Check sheet for the modelled part. Datum: model origin and axes. Units: mm. A direction names the side the tool comes from. Round coordinates to 2 decimals unless told otherwise and drop trailing zeros. Loops run counter-clockwise (first coordinate to the right, second up) from the corner with the lowest first, then second, coordinate; pieces in that order, holes last. Notation, with made-up numbers: (2, -13.75) -> (30, -13.75) arc R10 ccw to (30, 5.25) -> close; hole circle Ø4 at (62.5, -29). An arc over 180 degrees is marked (long way). One line per item, written item: value. Start each with the question number.
1. Material ranges on L1, parallel to X at y = 3.75, z = 1.4; L2, parallel to Y at x = 3.5, z = 1.75; L3, parallel to Y at x = 5, z = 4.8, recorded low to high.
2. Cross-section at C-C on y = 3. Record the cut outline in (x, z), then the cut area to 3 significant figures.
3. Release check for a two-part mould opening along X. For faces 6 (the face through (7, 2.25, 5)), 7 (the face through (0.301, 3.465, 5.715)), 8 (the face through (7, 0, 2)) record: +X half, -X half, draft (parallel to the pull), parting line (faces both ways), or undercut.
4. Cross-section at B-B on x = 11. Record the cut outline in (y, z).
5. Cross-section at D-D on x = 2.5. Record the cut outline in (y, z), then the cut area to 3 significant figures.
6. Cross-section at A-A on z = 2.85. Record the cut outline in (x, y), then the cut area to 3 significant figures.
7. Set-up check for faces 1 (the face through (6.9, 3.75, 3.5)), 2 (the face through (13.699, 0.285, 2.535)), 3 (the face through (8.5, 6.5, 0.5)), 4 (the face through (1.67, 3, 5)), 5 (the face through (13, 3, 1)): record each of +Z, -Z, +X, -X, +Y, -Y from which the full face is reachable in a straight line by a thin tool's end or side.
8. Go/stop test with a flat-tipped pin: pin 1 (1.2 mm diameter, centred on x = 8.5, y = 3.5, fed in from +Z). Record where the tip stops, or that it passes through.
Autodesk Inventor part; units mm, degrees
ref_plane "YZ Plane" through (0, 0, 0) normal (1, 0, 0) x (0, 1, 0)
ref_plane "XZ Plane" through (0, 0, 0) normal (0, 1, 0) x (-1, 0, 0)
ref_plane "XY Plane" through (0, 0, 0) normal (0, 0, 1) x (1, 0, 0)
sketch "Sketch1" plane through (0, 0, 0) normal (0, 0, 1) x (1, 0, 0)
  line L0 (0, 0) -> (14, 0)
  line L1 (14, 0) -> (14, 7)
  line L2 (14, 7) -> (0, 7)
  line L3 (0, 7) -> (0, 0)
  dimension "d2" = 14
  dimension "d3" = 7
extrude "Extrusion1" add sketch "Sketch1" along normal blind 6
sketch "Sketch2" plane through (0, 0, 6) normal (0, 0, 1) x (1, 0, 0)
  line L0 (0, 7) -> (14, 0) construction
  line L1 (0, 0) -> (14, 7) construction
  line L2 (1.67, 4.75) -> (12.33, 4.75)
  line L3 (12.33, 4.75) -> (12.33, 2.25)
  line L4 (12.33, 2.25) -> (1.67, 2.25)
  line L5 (1.67, 2.25) -> (1.67, 4.75)
  line L6 (1.67, 4.75) -> (12.33, 2.25) construction
  line L7 (12.33, 4.75) -> (1.67, 2.25) construction
  point P0 (7, 3.5)
  dimension "d4" = 2.5
  dimension "d5" = 10.66
extrude "Extrusion3" cut sketch "Sketch2" against normal blind 2
sketch "Sketch3" plane through (0, 0, 4) normal (0, 0, 1) x (1, 0, 0)
  line L0 (1.67, 4.75) -> (12.33, 4.75)
  line L1 (1.67, 2.25) -> (1.67, 4.75)
  line L2 (12.33, 2.25) -> (1.67, 2.25)
  line L3 (12.33, 4.75) -> (12.33, 2.25)
  line L4 (2.67, 3.75) -> (11.33, 3.75)
  line L5 (11.33, 3.75) -> (11.33, 3.25)
  line L6 (11.33, 3.25) -> (2.67, 3.25)
  line L7 (2.67, 3.25) -> (2.67, 3.75)
  point P0 (0, 0)
  dimension "d10" = 1
  dimension "d11" = 1
  dimension "d12" = 1
  dimension "d13" = 1
extrude "Extrusion4" cut sketch "Sketch3" against normal blind 4 contours L4 L5 L6 L7
sketch "Sketch4" plane through (0, 0, 0) normal (0, 0, -1) x (-1, 0, 0)
  line L0 (-2.67, 3.75) -> (-2.67, 3.25)
  line L1 (-2.67, 3.25) -> (-11.33, 3.25)
  line L2 (-11.33, 3.25) -> (-11.33, 3.75)
  line L3 (-11.33, 3.75) -> (-2.67, 3.75)
  line L4 (0, 0) -> (-14, 0)
  line L5 (0, 7) -> (0, 0)
  line L6 (-14, 7) -> (0, 7)
  line L7 (-14, 0) -> (-14, 7)
  line L8 (-13, 6) -> (-1, 6)
  line L9 (-1, 6) -> (-1, 1)
  line L10 (-1, 1) -> (-13, 1)
  line L11 (-13, 1) -> (-13, 6)
  dimension "d16" = 1
  dimension "d17" = 1
  dimension "d18" = 1
  dimension "d19" = 1
extrude "Extrusion5" cut sketch "Sketch4" against normal blind 3 contours L8 L9 L10 L11
sketch "Sketch5" plane through (0, 7, 0) normal (0, 1, 0) x (1, 0, 0)
  line L0 (14, 0) -> (0, 0)
  line L1 (0, 0) -> (0, -6)
  line L2 (14, 0) -> (14, -6)
  line L3 (5.5, 0) -> (8.5, 0)
  line L4 (8.5, 0) -> (8.5, -1)
  line L5 (8.5, -1) -> (5.5, -1)
  line L6 (5.5, -1) -> (5.5, 0)
  dimension "d22" = 1
  dimension "d23" = 5.5
  dimension "d24" = 5.5
  dimension "d25" = 3
extrude "Extrusion6" cut sketch "Sketch5" against normal blind 1
fillet "Fillet1" radius 1 8 edges at (7, 0, 6) (14, 3.5, 6) (14, 0, 3) (7, 7, 6) (14, 7, 3) (0, 0, 3) (0, 3.5, 6) (0, 7, 3)
properties part number "cover" material "Titanium"
Taken from the geometry:
1. L1: x = 0 to 1, 13 to 14
1. L2: y = 0 to 1, 6 to 7
1. L3: y = 0 to 2.25, 4.75 to 7
2. outline: (0, 0) -> (1, 0) -> (1, 3) -> (13, 3) -> (13, 0) -> (14, 0) -> (14, 5) arc R1 ccw to (13, 6) -> (12.33, 6) -> (12.33, 4) -> (1.67, 4) -> (1.67, 6) -> (1, 6) arc R1 ccw to (0, 5) -> close
2. area: 26.3 mm2
3. face 6: undercut
3. face 7: -X half
3. face 8: draft
4. outline: (0, 0) -> (1, 0) -> (1, 3) -> (3.25, 3) -> (3.25, 4) -> (2.25, 4) -> (2.25, 6) -> (1, 6) arc R1 ccw to (0, 5) -> close; (3.75, 3) -> (6, 3) -> (6, 0) -> (7, 0) -> (7, 5) arc R1 ccw to (6, 6) -> (4.75, 6) -> (4.75, 4) -> (3.75, 4) -> close
5. outline: (0, 0) -> (1, 0) -> (1, 3) -> (6, 3) -> (6, 0) -> (7, 0) -> (7, 5) arc R1 ccw to (6, 6) -> (4.75, 6) -> (4.75, 4) -> (2.25, 4) -> (2.25, 6) -> (1, 6) arc R1 ccw to (0, 5) -> close
5. area: 21.6 mm2
6. outline: (0, 1) arc R1 ccw to (1, 0) -> (13, 0) arc R1 ccw to (14, 1) -> (14, 6) arc R1 ccw to (13, 7) -> (1, 7) arc R1 ccw to (0, 6) -> close; hole (1, 1) -> (13, 1) -> (13, 6) -> (1, 6) -> close
6. area: 37.1 mm2
7. face 1: +Z, -Z
7. face 2: +Z, -Z, +X, -Y
7. face 3: -Z, +Y
7. face 4: +Z
7. face 5: -Z
8. pin 1: stops at z = 4
